Read the model definition and answer for the solid it produces. Units are mm, in the model's axes. Face numbers are marked on the shaded views. A direction names the side the tool comes from. Give positions to 0.01 mm unless a question says otherwise; leave off trailing zeros. Order: outer loops, then holes, each group sorted by start corner. A loop starts at its lowest first (then second) coordinate and runs counter-clockwise, first axis right, second up.
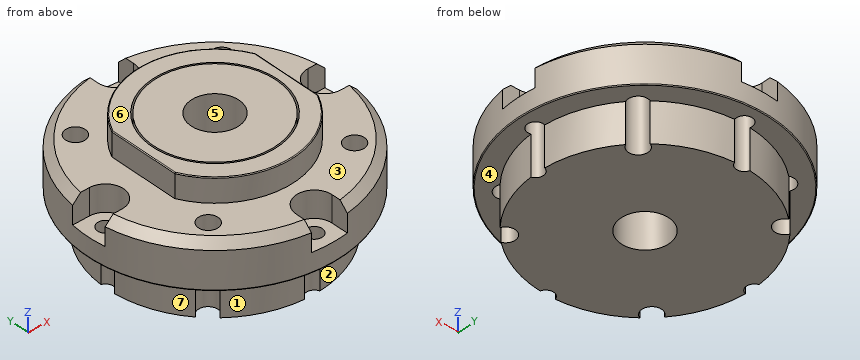
Autodesk Inventor part; units mm, degrees
ref_plane "YZ Plane" through (0, 0, 0) normal (1, 0, 0) x (0, 1, 0)
ref_plane "XZ Plane" through (0, 0, 0) normal (0, 1, 0) x (-1, 0, 0)
ref_plane "XY Plane" through (0, 0, 0) normal (0, 0, 1) x (1, 0, 0)
sketch "スケッチ1" plane through (0, 0, 0) normal (0, 0, 1) x (1, 0, 0)
  circle A0 centre (0, 0) radius 16
  dimension "d0" = 32
extrude "押し出し1" add sketch "スケッチ1" along normal blind 5.7
sketch "スケッチ2" plane through (0, 0, 0) normal (0, 0, -1) x (-1, 0, 0)
  circle A0 centre (0, 0) radius 13.5
  dimension "d3" = 27
extrude "押し出し2" add sketch "スケッチ2" along normal blind 5
sketch "スケッチ3" plane through (0, 0, 5.7) normal (0, 0, 1) x (1, 0, 0)
  circle A0 centre (0, 0) radius 10
  line L0 (-9, 4.3589) -> (9, 4.3589) construction
  line L1 (9, 4.3589) -> (9, -4.3589)
  line L2 (9, -4.3589) -> (-9, -4.3589) construction
  line L3 (-9, -4.3589) -> (-9, 4.3589)
  dimension "d6" = 20
  dimension "d7" = 18
extrude "押し出し3" add sketch "スケッチ3" along normal blind 3 contours L1 A0 L3
sketch "スケッチ4" plane through (0, 0, 8.7) normal (0, 0, 1) x (1, 0, 0)
  point P0 (0, 0)
  point P1 (0, 0)
hole "穴1" at (0, 0, 8.7) direction (0, 0, -1) diameter 6 end through all
sketch "スケッチ5" plane through (0, 0, 5.7) normal (0, 0, 1) x (1, 0, 0)
  circle A0 centre (0, 13.75) radius 2.25
  line L0 (-2.25, 13.75) -> (2.25, 13.75)
  line L1 (2.25, 13.75) -> (2.25, 16)
  line L2 (2.25, 16) -> (-2.25, 16)
  line L3 (-2.25, 16) -> (-2.25, 13.75)
  circle A1 centre (0, 0) radius 16
  circle A2 centre (-13.75, 0) radius 2.25
  line L4 (-13.75, -2.25) -> (-13.75, 2.25)
  line L5 (-13.75, 2.25) -> (-16, 2.25)
  line L6 (-16, 2.25) -> (-16, -2.25)
  line L7 (-16, -2.25) -> (-13.75, -2.25)
  circle A3 centre (0, -13.75) radius 2.25
  line L8 (2.25, -13.75) -> (-2.25, -13.75)
  line L9 (-2.25, -13.75) -> (-2.25, -16)
  line L10 (-2.25, -16) -> (2.25, -16)
  line L11 (2.25, -16) -> (2.25, -13.75)
  circle A4 centre (13.75, 0) radius 2.25
  line L12 (13.75, 2.25) -> (13.75, -2.25)
  line L13 (13.75, -2.25) -> (16, -2.25)
  line L14 (16, -2.25) -> (16, 2.25)
  line L15 (16, 2.25) -> (13.75, 2.25)
  point P0 (-15.841, -2.25)
  point P1 (-15.841, 2.25)
  point P2 (2.25, -15.841)
  point P3 (-2.25, -15.841)
  point P4 (15.841, -2.25)
  point P5 (15.841, 2.25)
  point P6 (2.25, 15.841)
  point P7 (-2.25, 15.841)
  dimension "d17" = 4.5
  dimension "d18" = 13.75
  dimension "d21" = 360
extrude "押し出し4" cut sketch "スケッチ5" against normal blind 3.3 contours L0 A0 | L3 A1 A0 | A0 L0 | A0 A1 L1 | L5 A2 A1 | A1 A4 L15 | A2 L7 A1 | A2 L4 | A2 L4 | A4 L12 | A1 L13 A4 | L12 A4 | L9 A3 A1 | A1 A3 L11 | A3 L8 | A3 L8
sketch "スケッチ6" plane through (0, 0, 2.4) normal (0, 0, 1) x (1, 0, 0)
  arc A0 (-2.25, 13.75) -> (2.25, 13.75) centre (0, 13.75) ccw
  arc A1 (13.75, 2.25) -> (13.75, -2.25) centre (13.75, 0) ccw
  arc A2 (2.25, -13.75) -> (-2.25, -13.75) centre (0, -13.75) ccw
  arc A3 (-13.75, -2.25) -> (-13.75, 2.25) centre (-13.75, 0) ccw
  point P0 (0, 0)
hole "穴2" at (0, 13.75, 2.4) at (13.75, 0, 2.4) at (0, -13.75, 2.4) at (-13.75, 0, 2.4) direction (0, 0, -1) diameter 2 end through all
sketch "スケッチ7" plane through (0, 0, 5.7) normal (0, 0, 1) x (1, 0, 0)
  line L0 (9.1924, 9.1924) -> (0, 0) construction
  line L1 (-22.4, 0) -> (22.4, 0)
  point P0 (-9.1924, 9.1924)
  point P1 (-9.1924, -9.1924)
  point P2 (9.1924, -9.1924)
  dimension "d32" = 45
  dimension "d33" = 13
  dimension "d36" = 360
hole "穴3" at (9.1924, 9.1924, 5.7) at (-9.1924, 9.1924, 5.7) at (-9.1924, -9.1924, 5.7) at (9.1924, -9.1924, 5.7) direction (0, 0, -1) diameter 2.459 end through all
sketch "スケッチ8" plane through (0, 0, 8.7) normal (0, 0, 1) x (1, 0, 0)
  circle A0 centre (0, 0) radius 3
  circle A1 centre (0, 0) radius 7.65
  circle A2 centre (0, 0) radius 7.85
  dimension "d45" = 15.3
  dimension "d46" = 15.7
extrude "押し出し5" cut sketch "スケッチ8" against normal up to surface (3 mm away) contours A2
chamfer "面取り1" distance 1 angle 45 4 edges at (11.3137, -11.3137, 5.7) (-11.3137, -11.3137, 5.7) (-11.3137, 11.3137, 5.7) (11.3137, 11.3137, 5.7)
fillet "フィレット1" radius 0.1 5 edges at (-16, 0, 0) (0, -10, 8.7) (9, 0, 8.7) (0, 10, 8.7) (-9, 0, 8.7)
properties part number "555_GearBox_FrontCover"
1) Consider L1, parallel to Y at x = 0, z = 6.35; L2, parallel to X at y = 0, z = 3.5; L3, parallel to X at y = -9.5, z = 3.5. Determine where each line is inside the solid, lowest interval first.
Final values:
L1: y = -10 to -7.85, -7.65 to -3, 3 to 7.65, 7.85 to 10
L2: x = -11.5 to -3, 3 to 11.5
L3: x = -12.87 to -10.38, -8 to 8, 10.38 to 12.87
2) A tool of negligible diameter and unlimited length cuts with its end or side. For the marked faces 1, 2, 3 and 4, from which of +Z, -Z, +X, -X, +Y, -Y can it reach the whole face along a straight path? Write none if from no direction.
Final values:
face 1: -Z, -X, -Y
face 2: -Z, +X, -Y
face 3: +Z
face 4: -Z
3) For a pull along Y with two mould halves and no side action, classify the marked faces 5, 6 and 7 as released by +Y, released by -Y, zero draft, split by the parting line, or undercut.
Final values:
face 5: undercut
face 6: zero draft
face 7: released by -Y
4) The part is cut by section A-A on z = -3.25. Determine the outline of the cut face in (x, y).
Final values:
outline: (-13.47, -0.96) arc R13.5 ccw to (-10.32, -8.7) arc R1.23 cw (long way) to (-8.7, -10.32) arc R13.5 ccw to (-0.96, -13.47) arc R1 cw to (0.96, -13.47) arc R13.5 ccw to (8.7, -10.32) arc R1.23 cw (long way) to (10.32, -8.7) arc R13.5 ccw to (13.47, -0.96) arc R1 cw to (13.47, 0.96) arc R13.5 ccw to (10.32, 8.7) arc R1.23 cw (long way) to (8.7, 10.32) arc R13.5 ccw to (0.96, 13.47) arc R1 cw to (-0.96, 13.47) arc R13.5 ccw to (-8.7, 10.32) arc R1.23 cw (long way) to (-10.32, 8.7) arc R13.5 ccw to (-13.47, 0.96) arc R1 cw to start; hole circle Ø6 at (0, 0)
5) Given pin 1 (3 mm diameter, centred on y = 11, z = -1, fed in from +X); pin 2 (1 mm diameter, centred on x = 15, z = 4, fed in from -Y); pin 3 (0.6 mm diameter, centred on y = -14.5, z = 4.5, fed in from +X), each flat-ended and moving along its own axis, determine where each tip first touches the part or whether it passes through.
Final values:
pin 1: stops at x = 12.53
pin 2: stops at y = -6.76
pin 3: stops at x = 7.37
6) The part is cut by section B-B on y = 0. Count the separate pieces of the cut face and the enclosed holes in it, and give its area (3 significant figures).
Final values:
separate pieces: 4
enclosed holes: 0
area: 241 mm2
